Source: CAD feature listing. Evaluate the final solid. Frame: model axes, mm. Face numbers are marked on the shaded views. A direction names the side the tool comes from. Give positions to 0.01 mm unless a question says otherwise; leave off trailing zeros. Order: outer loops, then holes, each group sorted by start corner. A loop starts at its lowest first (then second) coordinate and runs counter-clockwise, first axis right, second up.
from build123d import *

# Parameters (mm, degrees)
SKETCH1_W               = 355.6
SKETCH1_H               = 101.6
EXTRUDE1_DEPTH          = 25.4
SKETCH10_R              = 88.9
EXTRUDE2_DEPTH          = 25.4
F_10_CLEARANCE_HOLE1_D  = 5.1054
CIRPATTERN1_COUNT       = 3
F_3_8_CLEARANCE_HOLE2_D = 10.0838
LPATTERN1_COUNT         = 2
LPATTERN1_PITCH         = 15.24
LPATTERN1_COUNT_DIR2    = 2
LPATTERN1_PITCH_DIR2    = 196.596
F_3_8_CLEARANCE_HOLE1_D = 10.0838
LPATTERN2_COUNT         = 2
LPATTERN2_PITCH         = 304.8
LPATTERN2_COUNT_DIR2    = 2
LPATTERN2_PITCH_DIR2    = 50.8
LPATTERN3_COUNT         = 2
LPATTERN3_PITCH         = 7.62
LPATTERN3_COUNT_DIR2    = 2
LPATTERN3_PITCH_DIR2    = 91.44
FILLET2_R               = 12.7
CHAMFER1_SIZE           = 2.54


with BuildPart() as part:
    # Sketch1 → Extrude1 (new body)
    with BuildSketch(Plane.XY):
        Rectangle(SKETCH1_W, SKETCH1_H)
    extrude(amount=EXTRUDE1_DEPTH)

    # Sketch10 → Extrude2 (add)
    with BuildSketch(Plane.XY.offset(25.4)):
        Circle(SKETCH10_R)
    extrude(amount=-EXTRUDE2_DEPTH)

    # 10 Clearance Hole1 (through all)
    with Locations(Plane(origin=(0, 0, 0), x_dir=(-1, 0, 0), z_dir=(0, 0, -1))):
        with Locations((0, 76.2)):
            f_10_clearance_hole1 = Hole(F_10_CLEARANCE_HOLE1_D / 2)

    # CirPattern1: 10 Clearance Hole1 ×3 about axis
    cirpattern1_axis = Axis((0, 0, 0), (0, 0, 1))
    for i in range(1, CIRPATTERN1_COUNT):
        add(f_10_clearance_hole1.rotate(cirpattern1_axis, i * 360 / CIRPATTERN1_COUNT), mode=Mode.SUBTRACT)

    # 3_8 Clearance Hole2 (through all)
    with Locations(Plane.XY.offset(25.4)):
        with Locations((98.298, 7.62)):
            f_3_8_clearance_hole2 = Hole(F_3_8_CLEARANCE_HOLE2_D / 2)

    # LPattern1: 3_8 Clearance Hole2 2 × 2
    with Locations(*[(-j * LPATTERN1_PITCH_DIR2, -i * LPATTERN1_PITCH, 0) for i in range(LPATTERN1_COUNT) for j in range(LPATTERN1_COUNT_DIR2) if (i, j) != (0, 0)]):
        add(f_3_8_clearance_hole2, mode=Mode.SUBTRACT)

    # 3_8 Clearance Hole1 (through all)
    with Locations(Plane.XY.offset(25.4)):
        with Locations((-152.4, 25.4)):
            f_3_8_clearance_hole1 = Hole(F_3_8_CLEARANCE_HOLE1_D / 2)

    # LPattern2: 3_8 Clearance Hole1 2 × 2
    with Locations(*[(i * LPATTERN2_PITCH, -j * LPATTERN2_PITCH_DIR2, 0) for i in range(LPATTERN2_COUNT) for j in range(LPATTERN2_COUNT_DIR2) if (i, j) != (0, 0)]):
        add(f_3_8_clearance_hole1, mode=Mode.SUBTRACT)

    # Sketch8 → 1_4 _0.25_ Diameter Hole1 (revolve, cut)
    with BuildSketch(Plane(origin=(45.72, 3.81, 25.4), x_dir=(0, -1, 0), z_dir=(1, 0, 0))):
        Polygon((0, 0), (0, 27.307732465), (3.175, 25.4), (3.175, 0), align=None)
    f_1_4_0_25_diameter_hole1 = revolve(axis=Axis((45.72, 3.81, 31.75), (0, 0, -1)), mode=Mode.SUBTRACT)

    # LPattern3: 1_4 _0.25_ Diameter Hole1 2 × 2
    with Locations(*[(-j * LPATTERN3_PITCH_DIR2, -i * LPATTERN3_PITCH, 0) for i in range(LPATTERN3_COUNT) for j in range(LPATTERN3_COUNT_DIR2) if (i, j) != (0, 0)]):
        add(f_1_4_0_25_diameter_hole1, mode=Mode.SUBTRACT)

    # Fillet2
    fillet2_edges = [part.edges().sort_by_distance(p)[0] for p in [
        (72.955945611, 50.8, 12.7),
        (72.955945611, -50.8, 12.7),
        (-72.955945611, 50.8, 12.7),
        (-72.955945611, -50.8, 12.7),
    ]]
    fillet(fillet2_edges, radius=FILLET2_R)

    # Chamfer1
    chamfer1_edges = [part.edges().sort_by_distance(p)[0] for p in [
        (177.8, -50.8, 12.7),
        (-177.8, -50.8, 12.7),
        (-177.8, 50.8, 12.7),
        (177.8, 50.8, 12.7),
    ]]
    chamfer(chamfer1_edges, length=CHAMFER1_SIZE)


solid = part.part
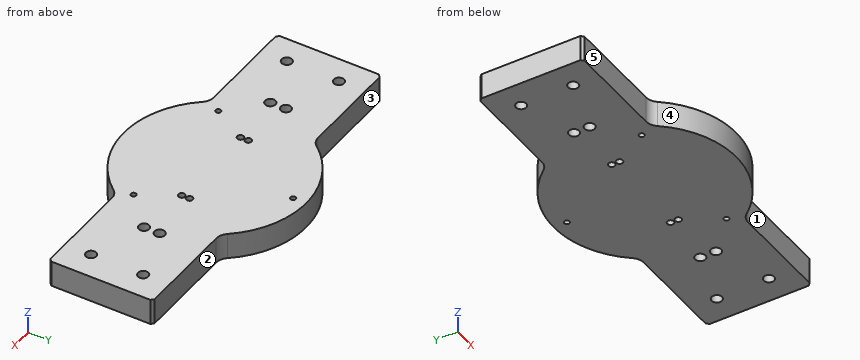
1) First-contact query: pin 1 Ø12.5 at (x, z) = (-107.5, 11) entering from -Y; pin 2 Ø1 at (x, z) = (85.5, 20.5) entering from +Y; pin 3 Ø8 at (x, y) = (152.4, 25.4) entering from +Z; pin 4 Ø5 at (x, z) = (-47.5, 15.5) entering from -Y. Flat tips, straight axial feed; report the tip coordinate or a pass-through.
Checks:
pin 1: stops at y = -50.8
pin 2: stops at y = 50.8
pin 3: passes through
pin 4: stops at y = -76.67
2) Section query C-C on x = -136.5. Output: boundary loops of the cut face in (y, z).
Checks:
outline: (-50.8, 0) - (50.8, 0) - (50.8, 25.4) - (-50.8, 25.4) - close
3) Ray query, L1, parallel to Y at x = 152.4, z = 6; L2, parallel to X at y = -25.5, z = 6; L3, parallel to Y at x = -48, z = 11. Return the intervals inside material, ascending.
Checks:
L1: y = -50.8 to -30.44, -20.36 to 20.36, 30.44 to 50.8
L2: x = -177.8 to -157.44, -147.36 to 147.36, 157.44 to 177.8
L3: y = -74.83 to -6.02, -1.6 to 1.6, 6.02 to 74.83
4) Reachability of the marked faces 1, 2, 3, 4 and 5 from +Z, -Z, +X, -X, +Y, -Y: full face, straight path, thin tool, end or side. Return the list, or none.
Checks:
face 1: +Z, -Z, +X, -Y
face 2: +Z, -Z, +X, +Y
face 3: +Z, -Z, -X, +Y
face 4: +Z, -Z, -Y
face 5: +Z, -Z, -X, -Y
5) Section query A-A on x = 152.4. Output: boundary loops of the cut face in (y, z).
Checks:
outline: (-50.8, 0) - (-30.44, 0) - (-30.44, 25.4) - (-50.8, 25.4) - close; (-20.36, 0) - (20.36, 0) - (20.36, 25.4) - (-20.36, 25.4) - close; (30.44, 0) - (50.8, 0) - (50.8, 25.4) - (30.44, 25.4) - close
6) Section query B-B on z = 14.75. State how many separate pieces and enclosed holes the cut face has, and give its area (3 significant figures).
Checks:
separate pieces: 1
enclosed holes: 15
area: 43,100 mm2
7) Section query D-D on x = 34. Output: boundary loops of the cut face in (y, z).
Checks:
outline: (-82.14, 0) - (82.14, 0) - (82.14, 25.4) - (-82.14, 25.4) - close
